Model file for the job. Use its own axes, mm. Face numbers are marked on the shaded views. A direction names the side the tool comes from. Round coordinates to 2 decimals unless told otherwise and drop trailing zeros. Order: outer loops, then holes, each group sorted by start corner. A loop starts at its lowest first (then second) coordinate and runs counter-clockwise, first axis right, second up. Notation, with made-up numbers: (88, 86.25) -> (122, 86.25) arc R24 cw to (122, 96.25) -> close; hole circle Ø4 at (89, 47). An arc over 180 degrees is marked (long way). Answer as CSV lines item,"result".
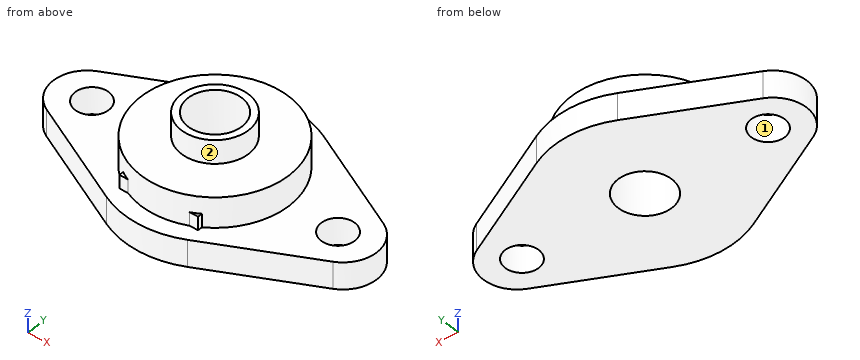
```python
from build123d import *

# Parameters (mm, degrees)
PAD_DEPTH       = 4
SKETCH001_R     = 2.5
POCKET_DEPTH    = 4.001
SKETCH002_R     = 11
PAD001_DEPTH    = 4.5
SKETCH003_R     = 5
PAD002_DEPTH    = 3.5
SKETCH004_R     = 4
POCKET001_DEPTH = 12.001
SKETCH005_W     = 11.67783
SKETCH005_H     = 2
PAD003_DEPTH    = 2


with BuildPart() as part:
    # Sketch → Pad (new body)
    with BuildSketch(Plane.XY):
        with BuildLine():
            ThreePointArc((21.236842, -4.471749), (24, 0), (21.236842, 4.471749))
            Line((21.236842, 4.471749), (6.039474, 12.073722))
            ThreePointArc((6.039474, 12.073722), (0, 13.5), (-6.039474, 12.073722))
            Line((-21.236842, 4.471749), (-6.039474, 12.073722))
            ThreePointArc((-21.236842, 4.471749), (-24, 0), (-21.236842, -4.471749))
            Line((-21.236842, -4.471749), (-6.039474, -12.073722))
            ThreePointArc((-6.039474, -12.073722), (0, -13.5), (6.039474, -12.073722))
            Line((6.039474, -12.073722), (21.236842, -4.471749))
        make_face()
    extrude(amount=PAD_DEPTH)

    # Sketch001 (on Face10 of Pad) → Pocket (cut, through all)
    with BuildSketch(Plane.XY.offset(4)):
        with Locations((-18.25, 0)):
            Circle(SKETCH001_R)
        with Locations((18.25, 0)):
            Circle(SKETCH001_R)
    extrude(amount=-POCKET_DEPTH, mode=Mode.SUBTRACT)

    # Sketch002 (on Face5 of Pocket) → Pad001 (join)
    with BuildSketch(Plane.XY.offset(4)):
        Circle(SKETCH002_R)
    extrude(amount=PAD001_DEPTH)

    # Sketch003 (on Face14 of Pad001) → Pad002 (join)
    with BuildSketch(Plane.XY.offset(8.5)):
        Circle(SKETCH003_R)
    extrude(amount=PAD002_DEPTH)

    # Sketch004 (on Face16 of Pad002) → Pocket001 (cut, through all)
    with BuildSketch(Plane.XY.offset(12)):
        Circle(SKETCH004_R)
    extrude(amount=-POCKET001_DEPTH, mode=Mode.SUBTRACT)

    # Sketch005 (on Face5 of Pocket001) → Pad003 (join)
    with BuildSketch(Plane.XY.offset(4)):
        with Locations((0, -9)):
            Rectangle(SKETCH005_W, SKETCH005_H)
    extrude(amount=PAD003_DEPTH)


solid = part.part
```
Q1. Saw through at C-C (z = 3). Write the cut outline in (x, y).
Checks:
outline,"(-21.24, -4.47) -> (-6.04, -12.07) arc R13.5 ccw to (6.04, -12.07) -> (21.24, -4.47) arc R5 ccw to (21.24, 4.47) -> (6.04, 12.07) arc R13.5 ccw to (-6.04, 12.07) -> (-21.24, 4.47) arc R5 ccw to start; hole circle Ø5 at (-18.25, 0); hole circle Ø8 at (0, 0); hole circle Ø5 at (18.25, 0)"
Q2. Flat gauge pins, fed straight in: pin 1 (0.5 mm diameter, centred on y = -9.5, z = 5, fed in from +X); pin 2 (6.5 mm diameter, centred on x = -18.25, y = 0, fed in from -Z); pin 3 (5 mm diameter, centred on y = -4, z = 8, fed in from +X); pin 4 (3 mm diameter, centred on y = 8, z = 7, fed in from +X). Where does each tip first touch, or does it go through?
Checks:
pin 1,"x = 5.95"
pin 2,"z = 0"
pin 3,"x = 10.9"
pin 4,"x = 8.87"
Q3. Saw through at A-A (x = 0). Write the cut outline in (y, z).
Checks:
outline,"(-13.5, 0) -> (-4, 0) -> (-4, 12) -> (-5, 12) -> (-5, 8.5) -> (-11, 8.5) -> (-11, 4) -> (-13.5, 4) -> close; (4, 0) -> (13.5, 0) -> (13.5, 4) -> (11, 4) -> (11, 8.5) -> (5, 8.5) -> (5, 12) -> (4, 12) -> close"
Q4. Saw through at D-D (x = 7.5). Write the cut outline in (y, z), plus the area to 3 significant figures.
Checks:
outline,"(-11.34, 0) -> (11.34, 0) -> (11.34, 4) -> (8.05, 4) -> (8.05, 8.5) -> (-8.05, 8.5) -> (-8.05, 4) -> (-11.34, 4) -> close"
area,"163 mm²"
Q5. Wall check: L1, parallel to Y at x = 0, z = 4.25; L2, parallel to Y at x = 0, z = 3; L3, parallel to X at y = 1.5, z = 1. Give the ranges that are in metal, low to high. Write a range as [from, to].
Checks:
L1,"[-11, -4], [4, 11]"
L2,"[-13.5, -4], [4, 13.5]"
L3,"[-23.77, -20.25], [-16.25, -3.71], [3.71, 16.25], [20.25, 23.77]"
Q6. Saw through at B-B (y = 0). Write the cut outline in (x, z).
Checks:
outline,"(-24, 0) -> (-20.75, 0) -> (-20.75, 4) -> (-24, 4) -> close; (-15.75, 0) -> (-4, 0) -> (-4, 12) -> (-5, 12) -> (-5, 8.5) -> (-11, 8.5) -> (-11, 4) -> (-15.75, 4) -> close; (4, 0) -> (15.75, 0) -> (15.75, 4) -> (11, 4) -> (11, 8.5) -> (5, 8.5) -> (5, 12) -> (4, 12) -> close; (20.75, 0) -> (24, 0) -> (24, 4) -> (20.75, 4) -> close"
Q7. Tool access for the marked faces 1 and 2: list every direction of +Z, -Z, +X, -X, +Y, -Y with a clear straight run to the whole face (end or side of a thin tool).
Checks:
face 1,"+Z, -Z"
face 2,"+Z"
